Input: part model. Units: mm. Frame: model coordinates. A direction names the side the tool comes from. Round coordinates to 2 decimals unless told otherwise and drop trailing zeros. Loops run counter-clockwise (first coordinate to the right, second up) from the corner with the lowest first, then second, coordinate; pieces in that order, holes last. Notation, with made-up numbers: (-25, 83.5) -> (7, 83.5) arc R23 ccw to (7, 115.5) -> close; hole circle Ø11 at (-6, 29.5). An arc over 180 degrees is marked (long way). Answer in a Markdown table with one row per item. Add a question column.
Q1. Section A-A, the plane y = -1.5. Output: boundary loops of the cut face in (x, z).
Q2. Section C-C, the plane y = -13.25. Output: boundary loops of the cut face in (x, z).
Q3. Pin query (flat end, axial travel): pin 1 (1 mm diameter, centred on y = 12.5, z = 5, fed in from -X); pin 2 (8 mm diameter, centred on x = 11, y = 26.5, fed in from -Z); pin 3 (0.6 mm diameter, centred on x = -15.5, z = 5.5, fed in from +Y). Return the tip coordinate at first contact, or that it passes through.
Q4. Section B-B, the plane x = -3. Output: boundary loops of the cut face in (y, z), and give its area (3 significant figures).
Q5. Mould query, pull axis Y, two halves, no side actions, for faces 1 (the face through (15.3, 13.3, 5)), 2 (the face through (-12, 24, 1.5)), 3 (the face through (0, 19.5, 3)). Classes: pulls with the +Y half, pulls with the -Y half, needs draft (parallel to the pull), parting line crosses it, or undercut.
Q6. Section D-D, the plane y = 14. Output: boundary loops of the cut face in (x, z), and give its area (3 significant figures).
Q7. Reachability of faces 4 (the face through (-32, -18, 3)), 5 (the face through (-16, -13, 4)), 6 (the face through (12, 24, 4.5)), 7 (the face through (-10, -14, 5)) from +Z, -Z, +X, -X, +Y, -Y: full face, straight path, thin tool, end or side. Return the list, or none.
Q8. Ray query, L1, parallel to Y at x = -13.6, z = 5.25; L2, parallel to Y at x = -18, z = 2.55; L3, parallel to Y at x = 11, z = 5.6. Return the intervals inside material, ascending. Write a range as from..to.
```python
from build123d import *

# Parameters (mm, degrees)
SKETCH_1_W          = 44
SKETCH_1_H          = 39
SKETCH_1_W_2        = 38
SKETCH_1_H_2        = 33
EXTRUDE_1_DEPTH     = 6
SKETCH_2_W          = 9
SKETCH_2_H          = 7
EXTRUDE_2_DEPTH     = 2
SKETCH_3_R          = 1.7
CUT_EXTRUDE_1_DEPTH = 30.669007398
EXTRUDE_3_DEPTH     = 1.5
SKETCH_5_W          = 10
SKETCH_5_H          = 3
EXTRUDE_4_DEPTH     = 6
FILLET_3_R          = 1
FILLET_4_R          = 2
SKETCH_6_R          = 1.7
CUT_EXTRUDE_2_DEPTH = 3


with BuildPart() as part:
    # 草图1 → 凸台-拉伸1 (new body)
    with BuildSketch(Plane.XY):
        Rectangle(SKETCH_1_W, SKETCH_1_H)
        Rectangle(SKETCH_1_W_2, SKETCH_1_H_2, mode=Mode.SUBTRACT)
    extrude(amount=EXTRUDE_1_DEPTH)

    # 草图2 → 凸台-拉伸2 (add)
    with BuildSketch(Plane.XY.offset(6)):
        with Locations((14.5, 13)):
            Rectangle(SKETCH_2_W, SKETCH_2_H)
        with Locations((-14.5, 13)):
            Rectangle(SKETCH_2_W, SKETCH_2_H)
        with Locations((-14.5, -13)):
            Rectangle(SKETCH_2_W, SKETCH_2_H)
        with Locations((14.5, -13)):
            Rectangle(SKETCH_2_W, SKETCH_2_H)
    extrude(amount=-EXTRUDE_2_DEPTH)

    # 草图3 → 切除-拉伸1 (cut, through all)
    with BuildSketch(Plane(origin=(0, 0, 4), x_dir=(-1, 0, 0), z_dir=(0, 0, -1))):
        with Locations((-13.6, 13.25)):
            Circle(SKETCH_3_R)
        with Locations(Location((13.6, 13.25, 0), (0, 0, 180))):
            Circle(SKETCH_3_R)
        with Locations((13.6, -13.25)):
            Circle(SKETCH_3_R)
        with Locations(Location((-13.6, -13.25, 0), (0, 0, 180))):
            Circle(SKETCH_3_R)
    extrude(amount=-CUT_EXTRUDE_1_DEPTH, mode=Mode.SUBTRACT)

    # 草图4 → 凸台-拉伸3 (add, symmetric)
    with BuildSketch(Plane(origin=(0, 0, 3), x_dir=(-1, 0, 0), z_dir=(0, 0, -1))):
        with BuildLine():
            Line((7.5, 19.5), (17.5, 19.5))
            add(Edge.make_bspline(
                [(7.5, 19.5), (12.5, 42.5), (17.5, 19.5)],
                knots=[0, 0, 0, 1, 1, 1], degree=2))
        make_face()
        with BuildLine():
            Line((-7.5, 19.5), (-17.5, 19.5))
            add(Edge.make_bspline(
                [(-7.5, 19.5), (-12.5, 42.5), (-17.5, 19.5)],
                knots=[0, 0, 0, 1, 1, 1], degree=2))
        make_face()
    extrude(amount=EXTRUDE_3_DEPTH, both=True)

    # 草图5 → 凸台-拉伸4 (add)
    with BuildSketch(Plane(origin=(0, 0, 0), x_dir=(-1, 0, 0), z_dir=(0, 0, -1))):
        with Locations((27, -18)):
            Rectangle(SKETCH_5_W, SKETCH_5_H)
        with Locations((-27, -18)):
            Rectangle(SKETCH_5_W, SKETCH_5_H)
    extrude(amount=-EXTRUDE_4_DEPTH)

    # 圆角3
    fillet_3_edges = [part.edges().sort_by_distance(p)[0] for p in [
        (-22, -16.5, 3),
        (-32, -18, 0),
        (-32, -18, 6),
        (22, -16.5, 3),
        (32, -18, 0),
        (32, -18, 6),
        (19, 16.5, 2),
        (10, 9.5, 5),
        (-19, 16.5, 2),
        (-10, 9.5, 5),
        (-19, -16.5, 2),
        (-10, -9.5, 5),
        (19, -16.5, 2),
        (10, -9.5, 5),
    ]]
    fillet(fillet_3_edges, radius=FILLET_3_R)

    # 圆角4
    fillet_4_edges = [part.edges().sort_by_distance(p)[0] for p in [
        (-22, 19.5, 3),
        (22, 19.5, 3),
    ]]
    fillet(fillet_4_edges, radius=FILLET_4_R)

    # 草图6 → 切除-拉伸2 (cut)
    with BuildSketch(Plane(origin=(0, -16.5, 0), x_dir=(1, 0, 0), z_dir=(0, 1, 0))):
        with Locations(Location((-27.5, -3, 0), (0, 0, 270))):
            Circle(SKETCH_6_R)
        with Locations(Location((27.5, -3, 0), (0, 0, 90))):
            Circle(SKETCH_6_R)
    extrude(amount=-CUT_EXTRUDE_2_DEPTH, mode=Mode.SUBTRACT)


solid = part.part
```
Answer block:
| question | item | result |
|---|---|---|
| 1 | outline | (-22, 0) -> (-19, 0) -> (-19, 6) -> (-22, 6) -> close; (19, 0) -> (22, 0) -> (22, 6) -> (19, 6) -> close |
| 2 | outline | (-22, 0) -> (-19, 0) -> (-19, 4) -> (-15.3, 4) -> (-15.3, 6) -> (-22, 6) -> close; (-11.9, 4) -> (-10, 4) -> (-10, 6) -> (-11.9, 6) -> close; (10, 4) -> (11.9, 4) -> (11.9, 6) -> (10, 6) -> close; (15.3, 4) -> (19, 4) -> (19, 0) -> (22, 0) -> (22, 6) -> (15.3, 6) -> close |
| 3 | pin 1 | x = -22 |
| 3 | pin 2 | z = 1.5 |
| 3 | pin 3 | y = 19.5 |
| 4 | outline | (-19.5, 0) -> (-16.5, 0) -> (-16.5, 6) -> (-19.5, 6) -> close; (16.5, 0) -> (19.5, 0) -> (19.5, 6) -> (16.5, 6) -> close |
| 4 | area | 36.0 mm^2 |
| 5 | face 1 | undercut |
| 5 | face 2 | needs draft |
| 5 | face 3 | pulls with the +Y half |
| 6 | outline | (-22, 0) -> (-19, 0) -> (-19, 4) -> (-15.13, 4) -> (-15.13, 6) -> (-22, 6) -> close; (-12.07, 4) -> (-10, 4) -> (-10, 6) -> (-12.07, 6) -> close; (10, 4) -> (12.07, 4) -> (12.07, 6) -> (10, 6) -> close; (15.13, 4) -> (19, 4) -> (19, 0) -> (22, 0) -> (22, 6) -> (15.13, 6) -> close |
| 6 | area | 59.8 mm^2 |
| 7 | face 4 | +Z, -Z, -X, +Y, -Y |
| 7 | face 5 | -Z |
| 7 | face 6 | +Z, +X, -X, +Y |
| 7 | face 7 | +Z, -Z |
| 8 | L1 | -19.5..-14.95, -11.55..-9.5, 9.5..11.55, 14.95..19.5 |
| 8 | L2 | -19.5..-16.5, 16.5..19.5 |
| 8 | L3 | -19.5..-9.5, 9.5..19.5 |
